Geometry check sheet. Reference: the model listing, model coordinates, mm. A direction names the side the tool comes from. Give positions to 0.01 mm unless a question says otherwise; leave off trailing zeros. Loops run counter-clockwise (first coordinate to the right, second up) from the corner with the lowest first, then second, coordinate; pieces in that order, holes last.
```python
from build123d import *

# Parameters (mm, degrees)
SKETCH1_W           = 88.3722
SKETCH1_H           = 86.137
BOSS_EXTRUDE1_DEPTH = 2
SKETCH2_W           = 3
SKETCH2_H           = 60
SKETCH2_W_2         = 60
SKETCH2_H_2         = 3
BOSS_EXTRUDE2_DEPTH = 10
FILLET1_R           = 5
FILLET2_R           = 5
FILLET3_R           = 1
CUT_EXTRUDE1_REACH  = 4
SKETCH3_W           = 60
SKETCH3_H           = 60


with BuildPart() as part:
    # Sketch1 → Boss-Extrude1 (new body)
    with BuildSketch(Plane.XY):
        with Locations((44.1861, 43.0685)):
            Rectangle(SKETCH1_W, SKETCH1_H)
    extrude(amount=BOSS_EXTRUDE1_DEPTH)

    # Sketch2 → Boss-Extrude2 (add)
    with BuildSketch(Plane.XY.offset(2)):
        with Locations((1.5, 43.0685)):
            Rectangle(SKETCH2_W, SKETCH2_H)
        with Locations((86.8722, 43.0685)):
            Rectangle(SKETCH2_W, SKETCH2_H)
        with Locations((44.1861, 1.5)):
            Rectangle(SKETCH2_W_2, SKETCH2_H_2)
        with Locations((44.1861, 84.637)):
            Rectangle(SKETCH2_W_2, SKETCH2_H_2)
    extrude(amount=BOSS_EXTRUDE2_DEPTH)

    # Fillet1
    fillet1_edges = [part.edges().sort_by_distance(p)[0] for p in [
        (0, 86.137, 1),
        (88.3722, 86.137, 1),
        (88.3722, 0, 1),
        (0, 0, 1),
    ]]
    fillet(fillet1_edges, radius=FILLET1_R)

    # Fillet2
    fillet2_edges = [part.edges().sort_by_distance(p)[0] for p in [
        (1.5, 13.0685, 2),
        (1.5, 73.0685, 2),
        (86.8722, 73.0685, 2),
        (86.8722, 13.0685, 2),
        (14.1861, 84.637, 2),
        (74.1861, 84.637, 2),
        (74.1861, 1.5, 2),
        (14.1861, 1.5, 2),
    ]]
    fillet(fillet2_edges, radius=FILLET2_R)

    # Fillet3
    fillet3_edges = [part.edges().sort_by_distance(p)[0] for p in [
        (0, 43.0685, 12),
        (1.5, 13.0685, 12),
        (3, 43.0685, 12),
        (1.5, 73.0685, 12),
        (88.3722, 43.0685, 12),
        (86.8722, 73.0685, 12),
        (85.3722, 43.0685, 12),
        (86.8722, 13.0685, 12),
        (14.1861, 84.637, 12),
        (44.1861, 83.137, 12),
        (74.1861, 84.637, 12),
        (44.1861, 86.137, 12),
        (44.1861, 0, 12),
        (74.1861, 1.5, 12),
        (44.1861, 3, 12),
        (14.1861, 1.5, 12),
    ]]
    fillet(fillet3_edges, radius=FILLET3_R)

    # Sketch3 → Cut-Extrude1 (cut, up to next)
    with BuildSketch(Plane.XY.offset(2), mode=Mode.PRIVATE) as cut_extrude1_sk1:
        with Locations((44.1861, 43.0685)):
            Rectangle(SKETCH3_W, SKETCH3_H)
    cut_extrude1_tool1 = extrude(cut_extrude1_sk1.sketch, amount=-CUT_EXTRUDE1_REACH, mode=Mode.PRIVATE) & part.part
    add(cut_extrude1_tool1.solids().sort_by_distance((44.1861, 43.0685, 2))[0], mode=Mode.SUBTRACT)


solid = part.part
```
1) Mould release check, pull along Y, two halves, no side actions. Record for faces 4 (the flat face through (44, 83.137, 6)), 5 (the flat face through (1, 13.068, 9)), 6 (the cylindrical face through (75.69, 84.658, 3.426)): +Y half, -Y half, draft (parallel to the pull), parting line (faces both ways), or undercut.
2) Sectioned sample at A-A on z = 8.75. Enter the section's corners in (x, y).
3) Sectioned sample at C-C on x = 45. Enter the section's corners in (y, z), plus the area to 3 significant figures.
4) Sectioned sample at D-D on z = 3. Enter the section's corners in (x, y), plus the area to 3 significant figures.
5) Depth check by flat-ended pin: P1, Ø0.9, axis at y = 85, z = 9.5, coming from the +X side; P2, Ø0.9, axis at y = 85, z = 10, coming from the -X side; P3, Ø3.5, axis at x = 1, z = 8.5, coming from the -Y side. Enter the tip coordinate at first touch or a pass-through.
6) Tool access check on faces 1 (the flat face through (14.186, 1, 9)), 2 (the flat face through (1, 73.068, 9)), 3 (the flat face through (74.186, 43, 1)). Record the directions out of +Z, -Z, +X, -X, +Y, -Y that give a thin tool (end or side, any length) a straight path to the whole face; none if there is none.
7) Sectioned sample at B-B on y = 29.5. Enter the section's corners in (x, z).
8) Scan lines: line 1 along X through (y, z) = (40, 6.5); line 2 along Y through (x, z) = (57.5, 5); line 3 along Y through (x, z) = (19, 0.5). Record each from-to range of solid material in increasing order.
Determined:
1. face 4: undercut
1. face 5: -Y half
1. face 6: draft
2. outline: (0, 13.07) - (3, 13.07) - (3, 73.07) - (0, 73.07) - close; (14.19, 0) - (74.19, 0) - (74.19, 3) - (14.19, 3) - close; (14.19, 83.14) - (74.19, 83.14) - (74.19, 86.14) - (14.19, 86.14) - close; (85.37, 13.07) - (88.37, 13.07) - (88.37, 73.07) - (85.37, 73.07) - close
3. outline: (0, 0) - (13.07, 0) - (13.07, 2) - (3, 2) - (3, 11) arc R1 ccw to (2, 12) - (1, 12) arc R1 ccw to (0, 11) - close; (73.07, 0) - (86.14, 0) - (86.14, 11) arc R1 ccw to (85.14, 12) - (84.14, 12) arc R1 ccw to (83.14, 11) - (83.14, 2) - (73.07, 2) - close
3. area: 111 mm2
4. outline: (0, 11.07) - (3, 11.07) - (3, 75.07) - (0, 75.07) - close; (12.19, 0) - (76.19, 0) - (76.19, 3) - (12.19, 3) - close; (12.19, 83.14) - (76.19, 83.14) - (76.19, 86.14) - (12.19, 86.14) - close; (85.37, 11.07) - (88.37, 11.07) - (88.37, 75.07) - (85.37, 75.07) - close
4. area: 768 mm2
5. P1: stops at x = 74.19
5. P2: stops at x = 14.19
5. P3: stops at y = 13.06
6. face 1: +Z, -X, +Y, -Y
6. face 2: +Z, +X, -X, +Y
6. face 3: +Z, -Z
7. outline: (0, 0) - (14.19, 0) - (14.19, 2) - (3, 2) - (3, 11) arc R1 ccw to (2, 12) - (1, 12) arc R1 ccw to (0, 11) - close; (74.19, 0) - (88.37, 0) - (88.37, 11) arc R1 ccw to (87.37, 12) - (86.37, 12) arc R1 ccw to (85.37, 11) - (85.37, 2) - (74.19, 2) - close
8. line 1: x = 0 to 3, 85.37 to 88.37
8. line 2: y = 0 to 3, 83.14 to 86.14
8. line 3: y = 0 to 13.07, 73.07 to 86.14
